The model under review builds one solid part; all positions refer to its coordinate system, in mm. Face numbers are marked on the shaded views. Round coordinates to 2 decimals unless told otherwise and drop trailing zeros. Write each loop counter-clockwise with the first axis right and the second up, starting at its lowest first coordinate (ties: lowest second). Pieces come first, ordered by that corner, then holes. Notation, with made-up numbers: (66, 86.25) - (122, 86.25) arc R30 cw to (122, 122.25) - close; hole circle Ø6 at (-35.5, 17.5). An arc over 180 degrees is marked (long way). Return JSON: item names as keys, results as strings.
Autodesk Inventor part; units mm, degrees
ref_plane "YZ Plane" through (0, 0, 0) normal (1, 0, 0) x (0, 1, 0)
ref_plane "XZ Plane" through (0, 0, 0) normal (0, 1, 0) x (-1, 0, 0)
ref_plane "XY Plane" through (0, 0, 0) normal (0, 0, 1) x (1, 0, 0)
sketch "スケッチ1" plane through (0, 0, 0) normal (1, 0, 0) x (0, 1, 0)
  circle A0 centre (0, 0) radius 17
  dimension "d0" = 34
extrude "押し出し1" add sketch "スケッチ1" along normal blind 5
sketch "スケッチ2" plane through (5, 0, 0) normal (1, 0, 0) x (0, 0, -1)
  circle A0 centre (0, 0) radius 13.5
  circle A1 centre (0, 0) radius 12.23
  line L0 (0, 0) -> (0, 13.5)
  line L1 (0, 0) -> (6.115, 10.5915)
  point P0 (-11.6913, 6.75)
  point P1 (-11.6913, -6.75)
  point P2 (0, -13.5)
  point P3 (11.6913, -6.75)
  point P4 (11.6913, 6.75)
  point P5 (-6.115, 10.5915)
  point P6 (-12.23, 0)
  point P7 (-6.115, -10.5915)
  point P8 (6.115, -10.5915)
  point P9 (12.23, 0)
  dimension "d3" = 27
  dimension "d4" = 24.46
  dimension "d5" = 30
  dimension "d8" = 360
  dimension "d12" = 360
hole "穴1" at (5, 13.5, 0) at (5, 6.75, 11.6913) at (5, -6.75, 11.6913) at (5, -13.5, 0) at (5, -6.75, -11.6913) at (5, 6.75, -11.6913) at (5, 10.5915, -6.115) at (5, 10.5915, 6.115) at (5, 0, 12.23) at (5, -10.5915, 6.115) at (5, 0, -12.23) at (5, -10.5915, -6.115) direction (-1, 0, 0) diameter 3.1 end through all
sketch "スケッチ3" plane through (5, 0, 0) normal (1, 0, 0) x (0, 0, -1)
  circle A0 centre (0, 0) radius 9
  dimension "d21" = 18
extrude "押し出し2" cut sketch "スケッチ3" against normal blind 5
properties part number "link2part6" material "アルミニウム 6061"
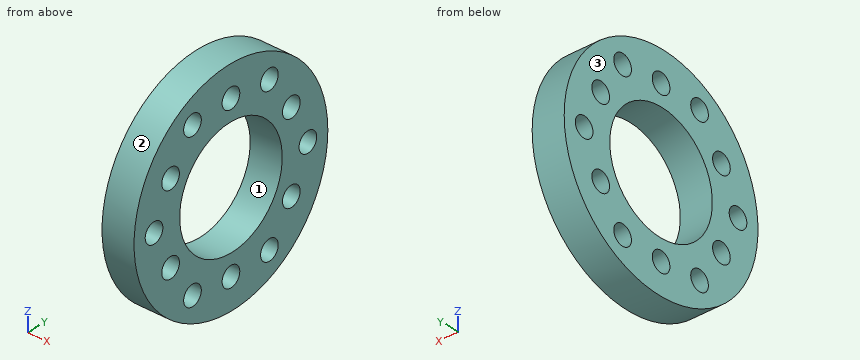
(1) Mouldability with a two-part tool opening along Z and no side actions: class the marked faces 1, 2 and 3 as released by +Z, released by -Z, zero draft, split by the parting line, or undercut.
Filled in:
{"face 1": "undercut", "face 2": "split by the parting line", "face 3": "zero draft"}
(2) Add section B-B (z = 12.5). Write out the cut boundary in (x, y), plus the area to 3 significant figures.
Filled in:
{"outline": "(0, -11.52) - (5, -11.52) - (5, -8.07) - (0, -8.07) - close; (0, -5.43) - (5, -5.43) - (5, -1.53) - (0, -1.53) - close; (0, 1.53) - (5, 1.53) - (5, 5.43) - (0, 5.43) - close; (0, 8.07) - (5, 8.07) - (5, 11.52) - (0, 11.52) - close", "area": "73.5 mm2"}
(3) Add section C-C (y = -10). Write out the cut boundary in (x, z).
Filled in:
{"outline": "(0, -13.75) - (5, -13.75) - (5, -7.55) - (0, -7.55) - close; (0, -4.68) - (5, -4.68) - (5, 4.68) - (0, 4.68) - close; (0, 7.55) - (5, 7.55) - (5, 13.75) - (0, 13.75) - close"}
(4) Wall thickness on line 1 (Z direction, x = 1.4, y = -8); line 2 (Y direction, x = 2.75, z = 13); line 3 (Y direction, x = 0.9, z = 12.5): over which ranges is each line inside the solid? List them lowest first.
Filled in:
{"line 1": "z = -15 to -12.61, -10.77 to -4.12, 4.12 to 10.77, 12.61 to 15", "line 2": "y = -10.95 to -7.58, -5.92 to -1.35, 1.35 to 5.92, 7.58 to 10.95", "line 3": "y = -11.52 to -8.07, -5.43 to -1.53, 1.53 to 5.43, 8.07 to 11.52"}
(5) Add section A-A (y = -3.5). Write out the cut boundary in (x, z).
Filled in:
{"outline": "(0, -16.64) - (5, -16.64) - (5, -8.29) - (0, -8.29) - close; (0, 8.29) - (5, 8.29) - (5, 16.64) - (0, 16.64) - close"}
(6) Clearance check with flat-ended pins moving along their axes: pin 1 Ø4 at (y, z) = (10.59, -6.12) entering from +X; pin 2 Ø2 at (x, z) = (2, 13) entering from +Y; pin 3 Ø1 at (x, z) = (2.5, 1.5) entering from +Y. State where each tip first meets the part, or that it passes through.
Filled in:
{"pin 1": "stops at x = 5", "pin 2": "stops at y = 12.04", "pin 3": "stops at y = 16.97"}
(7) Add section D-D (x = 2.05). Give the number of separate pieces and of enclosed holes in the cut face, plus the area to 3 significant figures.
Filled in:
{"separate pieces": "1", "enclosed holes": "13", "area": "563 mm2"}
